Part print with two shaded views. Sizes in mm from the minimum x, y, z corner. A direction names the side the tool comes from. Coordinates: 2 decimals unless noted, no trailing zeros. Loops run counter-clockwise (first coordinate to the right, second up) from the corner with the lowest first, then second, coordinate; pieces in that order, holes last.
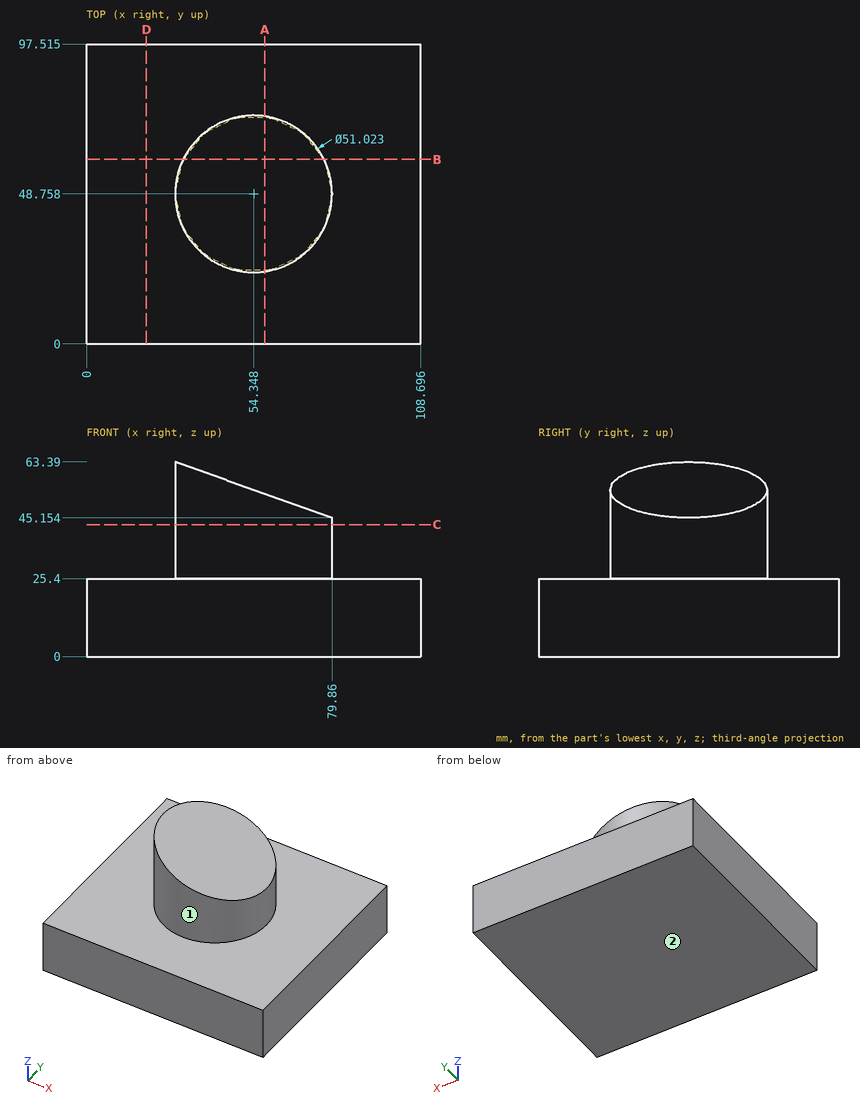
Q1. Slice it at A-A (x = 58). List the corners of the cut face in (y, z) (1 decimal).
Answers:
outline: (0, 0) - (97.5, 0) - (97.5, 25.4) - (74, 25.4) - (74, 53) - (23.5, 53) - (23.5, 25.4) - (0, 25.4) - close
Q2. Flat gauge pins, fed straight in: P1, Ø8, axis at x = 43, z = 39.5, coming from the +Y side; P2, Ø12, axis at x = 78.5, z = 13, coming from the -Y side; P3, Ø10, axis at x = 14.5, y = 12.5, coming from the +Z side; P4, Ø4, axis at y = 24.5, z = 55, coming from the -X side. Where does each tip first touch, or does it go through?
Answers:
P1: stops at y = 73.19
P2: stops at y = 0
P3: stops at z = 25.4
P4: stops at x = 41.88
Q3. Slice it at B-B (y = 60). List the corners of the cut face in (x, z), and give its area (3 significant figures).
Answers:
outline: (0, 0) - (108.7, 0) - (108.7, 25.4) - (77.25, 25.4) - (77.25, 46.09) - (31.45, 62.46) - (31.45, 25.4) - (0, 25.4) - close
area: 4,080 mm2
Q4. Drill centre lines: line 1 (Z direction, x = 19, y = 45); line 2 (X direction, y = 49.5, z = 29); line 3 (Y direction, x = 72, z = 38) (1 decimal). Where is each one in solid material? Low to high.
Answers:
line 1: z = 0 to 25.4
line 2: x = 28.85 to 79.85
line 3: y = 30.3 to 67.2
Q5. Slice it at C-C (z = 43). List the corners of the cut face in (x, y), and give its area (3 significant figures).
Answers:
outline: circle Ø51.02 at (54.35, 48.76)
area: 2,040 mm2
Q6. Slice it at D-D (x = 19.5). List the corners of the cut face in (y, z) (1 decimal).
Answers:
outline: (0, 0) - (97.5, 0) - (97.5, 25.4) - (0, 25.4) - close
Q7. Which spindle directions (+Z, -Z, +X, -X, +Y, -Y) get a long thin tool onto all of the face, cutting with end or side? Do the marked faces 1 and 2. Say none if no direction does.
Answers:
face 1: +Z
face 2: -Z, +X, -X, +Y, -Y
